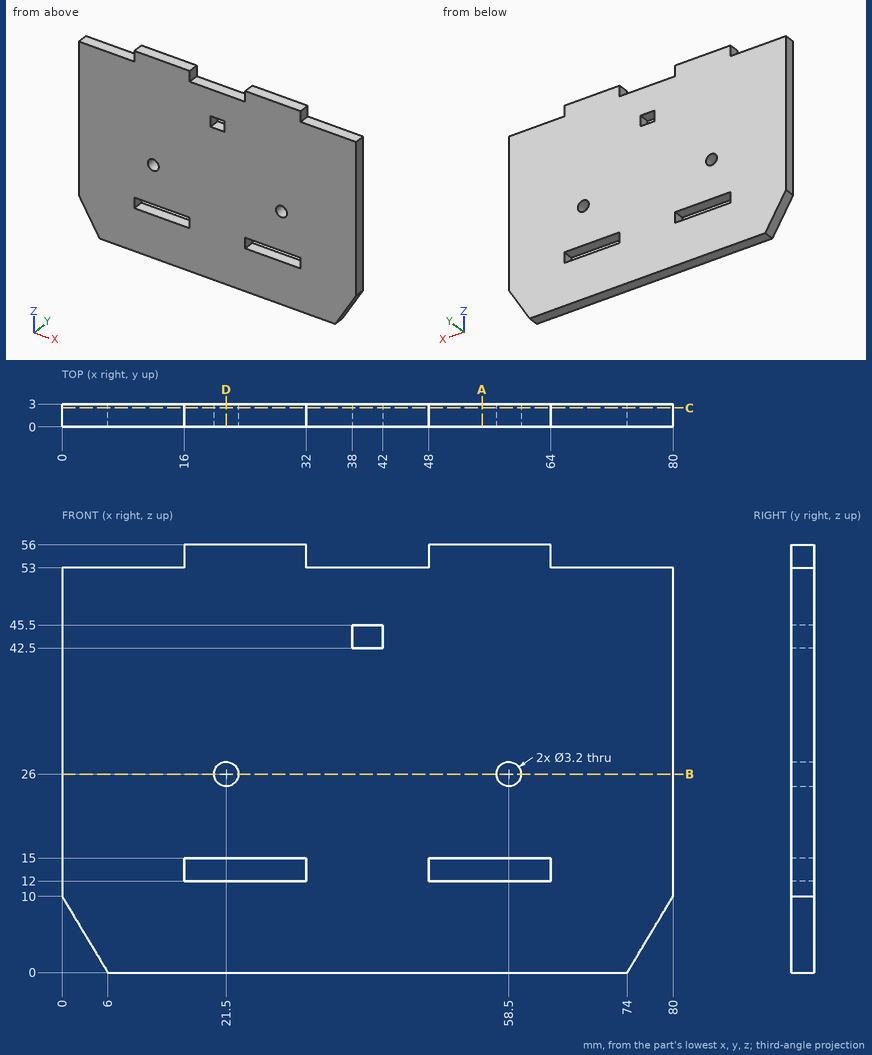
Job drawing, mm, ordinate dimensions from the low corner. One solid piece. Coordinates: 2 decimals unless noted, no trailing zeros. Order: outer loops, then holes, each group sorted by start corner. A loop starts at its lowest first (then second) coordinate and runs counter-clockwise, first axis right, second up. Notation, with made-up numbers: (34, -7) -> (48, -7) arc R26 cw to (48, 22) -> close; hole circle Ø7 at (-40, 55). An arc over 180 degrees is marked (long way). Return JSON: item names as keys, results as strings. Group by question number.
Item 1: Wall check: line 1 along X through (y, z) = (1.4, 26); line 2 along Z through (x, y) = (58.5, 1.4); line 3 along X through (y, z) = (1.05, 14). Give the ranges that are in metal, low to high. Write a range as [from, to].
Item 2: Flat gauge pins, fed straight in: P1, Ø1.5, axis at x = 40.5, y = 2, coming from the -Z side; P2, Ø1.5, axis at y = 2, z = 54, coming from the -X side; P3, Ø1.5, axis at x = 72, y = 1.5, coming from the +Z side; P4, Ø1.5, axis at y = 1.5, z = 54.5, coming from the +X side. Where does each tip first touch, or does it go through?
Item 3: Saw through at D-D on x = 21.5. Write the cut outline in (y, z).
Item 4: Saw through at B-B on z = 26. Write the cut outline in (x, y).
Item 5: Saw through at A-A on x = 55. Write the cut outline in (y, z), then the cut area to 3 significant figures.
Item 6: Saw through at C-C on y = 2.5. Write the cut outline in (x, z), then the cut area to 3 significant figures.
Values found:
{
 "1": {"line 1": "x = [0, 19.9], [23.1, 56.9], [60.1, 80]", "line 2": "z = [0, 12], [15, 24.4], [27.6, 56]", "line 3": "x = [0, 16], [32, 48], [64, 80]"},
 "2": {"P1": "stops at z = 0", "P2": "stops at x = 16", "P3": "stops at z = 53", "P4": "stops at x = 64"},
 "3": {"outline": "(0, 0) -> (3, 0) -> (3, 12) -> (0, 12) -> close; (0, 15) -> (3, 15) -> (3, 24.4) -> (0, 24.4) -> close; (0, 27.6) -> (3, 27.6) -> (3, 56) -> (0, 56) -> close"},
 "4": {"outline": "(0, 0) -> (19.9, 0) -> (19.9, 3) -> (0, 3) -> close; (23.1, 0) -> (56.9, 0) -> (56.9, 3) -> (23.1, 3) -> close; (60.1, 0) -> (80, 0) -> (80, 3) -> (60.1, 3) -> close"},
 "5": {"outline": "(0, 0) -> (3, 0) -> (3, 12) -> (0, 12) -> close; (0, 15) -> (3, 15) -> (3, 56) -> (0, 56) -> close", "area": "159 mm2"},
 "6": {"outline": "(0, 10) -> (6, 0) -> (74, 0) -> (80, 10) -> (80, 53) -> (64, 53) -> (64, 56) -> (48, 56) -> (48, 53) -> (32, 53) -> (32, 56) -> (16, 56) -> (16, 53) -> (0, 53) -> close; hole (16, 12) -> (32, 12) -> (32, 15) -> (16, 15) -> close; hole circle Ø3.2 at (21.5, 26); hole (38, 42.5) -> (42, 42.5) -> (42, 45.5) -> (38, 45.5) -> close; hole (48, 12) -> (64, 12) -> (64, 15) -> (48, 15) -> close; hole circle Ø3.2 at (58.5, 26)", "area": "4,150 mm2"}
}
